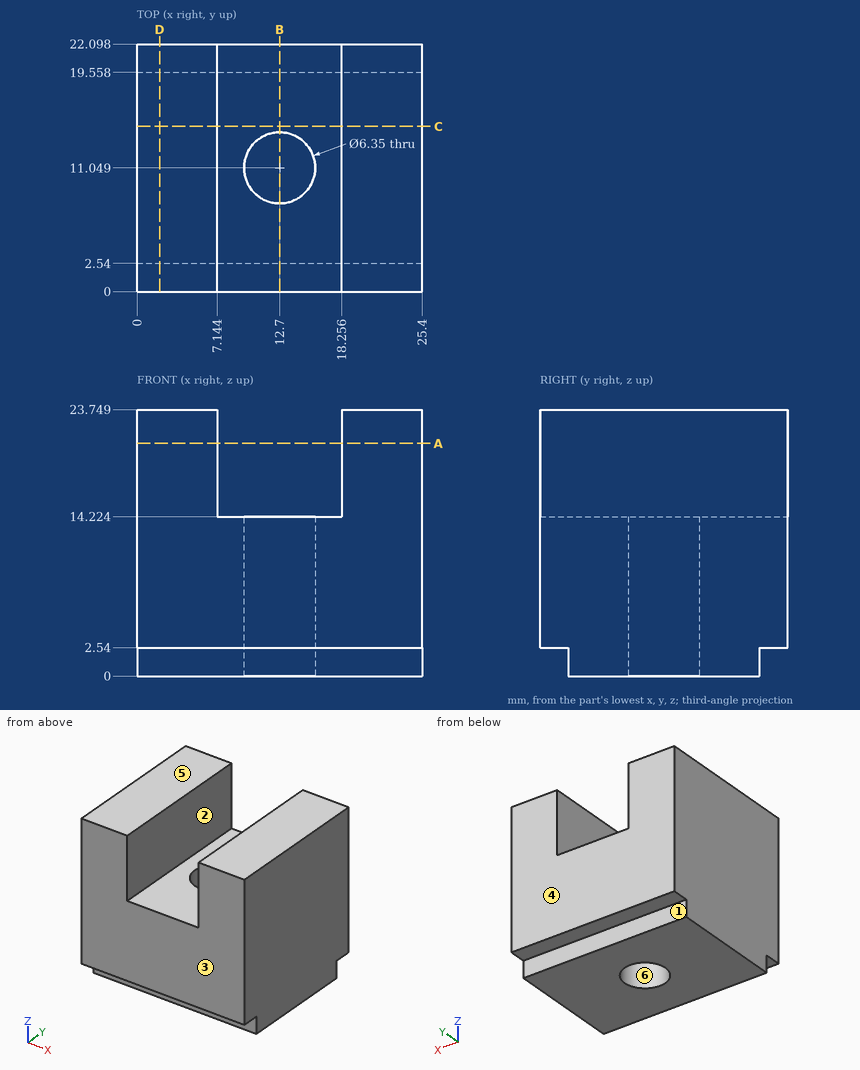
Input: dimensioned drawing with shaded views. Units: mm. Origin: part minimum x, y, z. A direction names the side the tool comes from. Give positions to 0.01 mm unless a question says otherwise; leave off trailing zeros. Write each loop counter-clockwise with the first axis right and the second up, starting at its lowest first coordinate (ties: lowest second). Pieces come first, ordered by that corner, then holes.
1. First-contact query: pin 1 (2 mm diameter, centred on x = 8, y = 1, fed in from -Z); pin 2 (6 mm diameter, centred on x = 14, y = 3.5, fed in from +Z); pin 3 (0.8 mm diameter, centred on x = 11.5, z = 1.5, fed in from +Y); pin 4 (5.5 mm diameter, centred on x = 12.7, y = 11.049, fed in from +Z). Flat tips, straight axial feed; report the tip coordinate or a pass-through.
2. Section query B-B (x = 12.7). Return the cut outline in (y, z), then the cut area to 3 significant figures.
3. Section query D-D (x = 2). Return the cut outline in (y, z), then the cut area to 3 significant figures.
4. Access query for the marked faces 1, 2 and 3. Directions: +Z, -Z, +X, -X, +Y, -Y. A direction counts if a zero-diameter tool reaches every point of the face in a straight line with its end or side. Return the directions, or none.
5. Pull-direction query (Y, two-part tool) for the marked faces 4, 5 and 6; classes: +Y half, -Y half, draft (parallel to the pull), parting line (faces both ways), or undercut.
6. Section query C-C (y = 14.75). Return the cut outline in (x, z).
7. Material intervals for line 1 along Y through (x, z) = (12.7, 6); line 2 along X through (y, z) = (18.5, 15); line 3 along Z through (x, y) = (9.5, 20.25), sorted ascending.
8. Section query A-A (z = 20.75). Return the cut outline in (x, y), then the cut area to 3 significant figures.
Output values:
1. pin 1: stops at z = 2.54
1. pin 2: stops at z = 14.22
1. pin 3: stops at y = 19.56
1. pin 4: passes through
2. outline: (0, 2.54) - (2.54, 2.54) - (2.54, 0) - (7.87, 0) - (7.87, 14.22) - (0, 14.22) - close; (14.22, 0) - (19.56, 0) - (19.56, 2.54) - (22.1, 2.54) - (22.1, 14.22) - (14.22, 14.22) - close
2. area: 211 mm2
3. outline: (0, 2.54) - (2.54, 2.54) - (2.54, 0) - (19.56, 0) - (19.56, 2.54) - (22.1, 2.54) - (22.1, 23.75) - (0, 23.75) - close
3. area: 512 mm2
4. face 1: -Z, +X, -X, +Y
4. face 2: +Z, +Y, -Y
4. face 3: +Z, -Z, +X, -X, -Y
5. face 4: +Y half
5. face 5: draft
5. face 6: undercut
6. outline: (0, 0) - (25.4, 0) - (25.4, 23.75) - (18.26, 23.75) - (18.26, 14.22) - (7.14, 14.22) - (7.14, 23.75) - (0, 23.75) - close
7. line 1: y = 0 to 7.87, 14.22 to 22.1
7. line 2: x = 0 to 7.14, 18.26 to 25.4
7. line 3: z = 2.54 to 14.22
8. outline: (0, 0) - (7.14, 0) - (7.14, 22.1) - (0, 22.1) - close; (18.26, 0) - (25.4, 0) - (25.4, 22.1) - (18.26, 22.1) - close
8. area: 316 mm2
